The listing builds one solid part. Answer for the finished solid, in the listing's coordinates (mm). A direction names the side the tool comes from. Round coordinates to 2 decimals unless told otherwise and drop trailing zeros. Loops run counter-clockwise (first coordinate to the right, second up) from the corner with the lowest first, then second, coordinate; pieces in that order, holes last. Notation, with made-up numbers: (23, 74) -> (50, 74) arc R24 cw to (50, 97) -> close; hole circle Ø7 at (16, 61.5). An arc over 180 degrees is marked (long way). Write each question's results on one line, items separated by ' | '. Start each with the question number.
(1) The part is cut by section D-D (x = 32). Determine the outline of the cut face in (y, z).
(2) Flat-ended cylindrical pins translate along their axes: pin 1 (6 mm diameter, centred on y = 16.5, z = -9, fed in from -X); pin 2 (5 mm diameter, centred on y = 6, z = -7, fed in from -X); pin 3 (1.9 mm diameter, centred on y = 18, z = 4.5, fed in from -X); pin 4 (1 mm diameter, centred on x = 21, y = 2.5, fed in from -Z). Find the tip coordinate at first contact, or state that the pin passes through.
(3) The part is cut by section A-A (x = 20). Determine the outline of the cut face in (y, z), plus the area to 3 significant figures.
(4) Determine the mould class of faces 1 (the face through (20, 15, -5)), 2 (the face through (21, 17.412, 5)), 3 (the face through (31, 0, -1)) for opening direction X: released by +X, released by -X, zero draft, split by the parting line, or undercut.
(5) Straight lines are drawn through the part: probe 1 along Z at (x, y) = (36, 1.75); probe 2 along Z at (x, y) = (31, 3); probe 3 along X at (y, z) = (18, 5). For each, find the intervals that lie inside material, in ascending order.
(6) For faces 4 (the face through (18.193, 19, 5)), 5 (the face through (20, 6, -18)), 6 (the face through (21.4, 15.2, 0)), determine the directions among +Z, -Z, +X, -X, +Y, -Y from which every point of the face is accessible in a straight line to the end or side of a thin tool.
(7) The part is cut by section C-C (y = 8.5). Determine the outline of the cut face in (x, z).
(8) The part is cut by section B-B (z = 8). Determine the outline of the cut face in (x, y), plus the area to 3 significant figures.
```python
from build123d import *

# Parameters (mm, degrees)
BOSS_EXTRUDE1_DEPTH     = 10
CUT_EXTRUDE1_DEPTH      = 12
CUT_EXTRUDE1_DEPTH_BACK = 19
SKETCH3_W               = 5
SKETCH3_H               = 4.533190639
BOSS_EXTRUDE2_DEPTH     = 10
BOSS_EXTRUDE3_DEPTH     = 8
CUT_EXTRUDE3_DEPTH      = 41


with BuildPart() as part:
    # Sketch2 → Boss-Extrude1 (new body)
    with BuildSketch(Plane.XY):
        with BuildLine():
            Line((0, 0), (40, 0))
            ThreePointArc((40, 0), (20, 20), (0, 0))
        make_face()
    extrude(amount=BOSS_EXTRUDE1_DEPTH)

    # Sketch3 → Cut-Extrude1 (cut, two sides: drawn at the far end of the back side and taken through both)
    with BuildSketch(Plane.XY.offset(10).offset(-CUT_EXTRUDE1_DEPTH_BACK)):
        with Locations((20.692849678, 19.678974606)):
            Rectangle(SKETCH3_W, SKETCH3_H)
    extrude(amount=CUT_EXTRUDE1_DEPTH + CUT_EXTRUDE1_DEPTH_BACK, mode=Mode.SUBTRACT)

    # Sketch4 → Boss-Extrude2 (add)
    with BuildSketch(Plane(origin=(0, 0, 0), x_dir=(-1, 0, 0), z_dir=(0, 0, -1))):
        with BuildLine():
            Line((-35, 0), (-5, 0))
            ThreePointArc((-5, 0), (-20, 15), (-35, 0))
        make_face()
    extrude(amount=BOSS_EXTRUDE2_DEPTH)

    # Sketch5 → Boss-Extrude3 (add)
    with BuildSketch(Plane(origin=(0, 0, -10), x_dir=(-1, 0, 0), z_dir=(0, 0, -1))):
        with BuildLine():
            Line((-30, 0), (-10, 0))
            ThreePointArc((-10, 0), (-20, 10), (-30, 0))
        make_face()
    extrude(amount=BOSS_EXTRUDE3_DEPTH)

    # Sketch6 → Cut-Extrude3 (cut)
    with BuildSketch(Plane(origin=(0, 0, -18), x_dir=(-1, 0, 0), z_dir=(0, 0, -1))):
        with BuildLine():
            Line((-25, 0), (-15, 0))
            ThreePointArc((-15, 0), (-20, 5), (-25, 0))
        make_face()
    extrude(amount=-CUT_EXTRUDE3_DEPTH, mode=Mode.SUBTRACT)


solid = part.part
```
Checked values:
1) outline: (0, -10) -> (9, -10) -> (9, 0) -> (16, 0) -> (16, 10) -> (0, 10) -> close
2) pin 1: stops at x = 13.46 | pin 2: stops at x = 5.41 | pin 3: stops at x = 9.55 | pin 4: passes through
3) outline: (5, -18) -> (10, -18) -> (10, -10) -> (15, -10) -> (15, 0) -> (17.41, 0) -> (17.41, 10) -> (5, 10) -> close | area: 264 mm2
4) face 1: split by the parting line | face 2: undercut | face 3: zero draft
5) probe 1: z = 0 to 10 | probe 2: z = -10 to 10 | probe 3: x = 11.28 to 18.19, 23.19 to 28.72
6) face 4: +Z, -Z, +Y | face 5: -Z, +X, -X, +Y, -Y | face 6: -Z, +Y
7) outline: (1.9, 0) -> (7.64, 0) -> (7.64, -10) -> (14.73, -10) -> (14.73, -18) -> (25.27, -18) -> (25.27, -10) -> (32.36, -10) -> (32.36, 0) -> (38.1, 0) -> (38.1, 10) -> (1.9, 10) -> close
8) outline: (0, 0) -> (15, 0) arc R5 cw to (25, 0) -> (40, 0) arc R20 ccw to (23.19, 19.74) -> (23.19, 17.41) -> (18.19, 17.41) -> (18.19, 19.92) arc R20 ccw to start | area: 576 mm2
